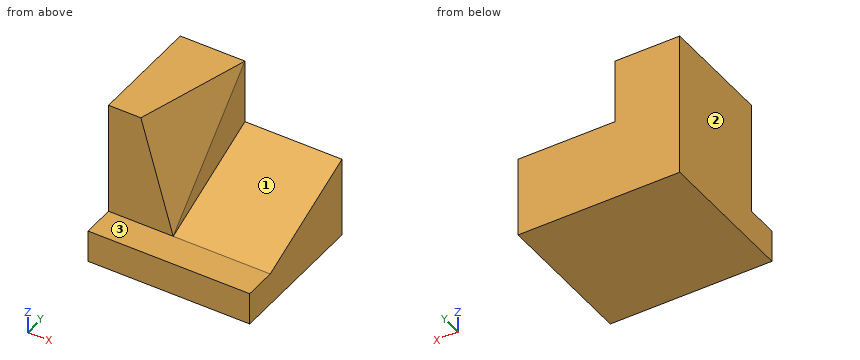
from build123d import *

# Parameters (mm, degrees)
F1_DEPTH = 10
F2_DEPTH = 4
F6_DEPTH = 7.9481941424


with BuildPart() as f1:
    # F0 (on Right) → F1 (new body)
    with BuildSketch(Plane.YZ):
        Polygon((0, 2), (0, 0), (9, 0), (9, 2), (2, 2), align=None)
        Polygon((2, 2), (9, 2), (9, 5), align=None)
    extrude(amount=F1_DEPTH)

    # F0 (on Right) → F2 (join)
    with BuildSketch(Plane.YZ):
        Polygon((2, 9), (2, 2), (9, 5), (9, 9), align=None)
    extrude(amount=F2_DEPTH)

    # F5 (on 3pt) → F6 (cut, through all)
    with BuildSketch(Plane(origin=(3.4385964912, -0.9824561404, 0.9824561404), x_dir=(-0.2547139161, -0.9642741111, -0.0727754046), z_dir=(-0.9271726499, 0.2649064714, -0.2649064714))):
        Polygon((-3.0929546961, 0.8241633837), (-3.0929546961, 8.104273273), (-10.3523013063, 7.5548310172), align=None)
    extrude(amount=-F6_DEPTH, mode=Mode.SUBTRACT)


solid = f1.part
Read the model definition and answer for the solid it produces. Units are mm, in the model's axes. Face numbers are marked on the shaded views. A direction names the side the tool comes from. Round coordinates to 2 decimals unless told otherwise and drop trailing zeros. Write each loop counter-clockwise with the first axis right and the second up, starting at its lowest first coordinate (ties: lowest second). Pieces come first, ordered by that corner, then holes.
1. The part is cut by section A-A, the plane x = 2.5. Determine the outline of the cut face in (y, z), then the cut area to 3 significant figures.
2. Straight lines are drawn through the part: L1, parallel to X at y = 7.5, z = 7.5; L2, parallel to Z at x = 6, y = 1.25; L3, parallel to X at y = 2.5, z = 5.75. For each, find the intervals that lie inside material, in ascending order.
3. Which of the six approach directions +Z, -Z, +X, -X, +Y, -Y give full straight-line access (tool end or side, diameter ignored) to the marked faces 1, 2 and 3?
4. The part is cut by section B-B, the plane z = 7.25. Determine the outline of the cut face in (x, y), then the cut area to 3 significant figures.
5. The part is cut by section D-D, the plane x = 8. Determine the outline of the cut face in (y, z).
6. The part is cut by section C-C, the plane y = 4.5. Determine the outline of the cut face in (x, z).
7. Given pin 1 Ø2 at (x, z) = (1, 6.5) entering from -Y; pin 2 Ø4 at (x, z) = (5.5, 7) entering from +Y; pin 3 Ø2 at (y, z) = (4.5, 6.5) entering from +X; pin 4 Ø2 at (y, z) = (4, 6.5) entering from +X, each flat-ended and moving along its own axis, determine where each tip first touches the part or whether it passes through.
Values:
1. outline: (0, 0) - (9, 0) - (9, 9) - (3.75, 9) - (2, 7.25) - (2, 2) - (0, 2) - close
1. area: 65.5 mm2
2. L1: x = 0 to 4
2. L2: z = 0 to 2
2. L3: x = 0 to 3.07
3. face 1: +Z, +X, -Y
3. face 2: +Z, -Z, -X, +Y, -Y
3. face 3: +Z, +X, -X, -Y
4. outline: (0, 2) - (2.5, 2) - (4, 7.25) - (4, 9) - (0, 9) - close
4. area: 24.1 mm2
5. outline: (0, 0) - (9, 0) - (9, 5) - (2, 2) - (0, 2) - close
6. outline: (0, 0) - (10, 0) - (10, 3.07) - (4, 3.07) - (4, 4.5) - (2.71, 9) - (0, 9) - close
7. pin 1: stops at y = 2
7. pin 2: stops at y = 9
7. pin 3: stops at x = 3.83
7. pin 4: stops at x = 3.69
